Source: CAD feature listing. Evaluate the final solid. Frame: model axes, mm. Face numbers are marked on the shaded views. A direction names the side the tool comes from. Round coordinates to 2 decimals unless told otherwise and drop trailing zeros. Loops run counter-clockwise (first coordinate to the right, second up) from the corner with the lowest first, then second, coordinate; pieces in that order, holes last. Notation, with made-up numbers: (75, -10) - (131, -10) arc R17 cw to (131, 12) - close; hole circle Ø7 at (60, 60.5). An arc over 180 degrees is marked (long way). Use CSV: the item, a comma, the result in double quotes. Start each with the question number.
from build123d import *

# Parameters (mm, degrees)
SKETCH1_R           = 15
SKETCH1_R_2         = 13
BOSS_EXTRUDE1_DEPTH = 13
SKETCH2_R           = 18
SKETCH2_R_2         = 13
BOSS_EXTRUDE2_DEPTH = 2
CHAMFER1_SIZE       = 1
SKETCH4_R           = 18
SKETCH4_R_2         = 16.05
BOSS_EXTRUDE3_DEPTH = 3.8


with BuildPart() as part:
    # Sketch1 → Boss-Extrude1 (new body)
    with BuildSketch(Plane.XY):
        Circle(SKETCH1_R)
        Circle(SKETCH1_R_2, mode=Mode.SUBTRACT)
    extrude(amount=BOSS_EXTRUDE1_DEPTH)

    # Sketch2 → Boss-Extrude2 (add)
    with BuildSketch(Plane.XY.offset(13)):
        Circle(SKETCH2_R)
        Circle(SKETCH2_R_2, mode=Mode.SUBTRACT)
    extrude(amount=BOSS_EXTRUDE2_DEPTH)

    # Chamfer1
    chamfer1_edges = [part.edges().sort_by_distance(p)[0] for p in [
        (-13, 0, 15),
    ]]
    chamfer(chamfer1_edges, length=CHAMFER1_SIZE)

    # Sketch4 → Boss-Extrude3 (add)
    with BuildSketch(Plane.XY.offset(15)):
        Circle(SKETCH4_R)
        with Locations(Location((0, 0, 0), (0, 0, 180))):
            Circle(SKETCH4_R_2, mode=Mode.SUBTRACT)
    extrude(amount=BOSS_EXTRUDE3_DEPTH)


solid = part.part
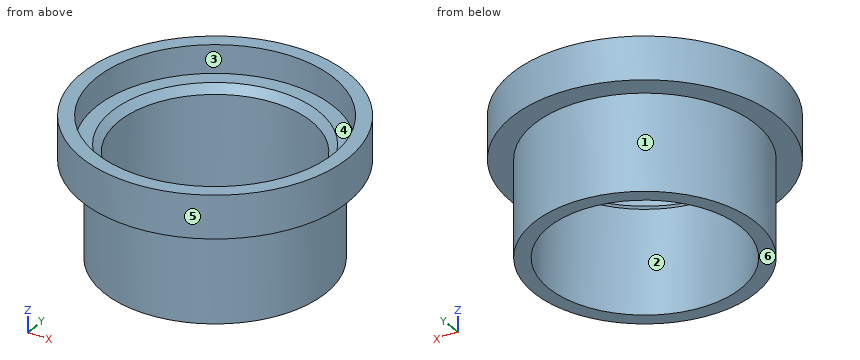
1. Section query C-C on z = 1.5. Return the cut outline in (x, y), and give its area (3 significant figures).
2. Contact query for flat-ended pins moving along their axis: P1, Ø10, axis at x = 12.5, y = -9, coming from the +Z side; P2, Ø2, axis at x = 1, z = 5, coming from the +Y side; P3, Ø1, axis at y = -5.5, z = 6.5, coming from the +X side; P4, Ø4, axis at y = -6.5, z = 10.5, coming from the -X side. Output: stop coordinate, or through.
3. Section query A-A on x = 0. Return the cut outline in (y, z).
4. Line query: line 1 along Y through (x, z) = (0, 7.5); line 2 along Y through (x, z) = (0, 17.15); line 3 along X through (y, z) = (-0.5, 12.5). Output: solid intervals per line, ascending.
5. Mould query, pull axis Y, two halves, no side actions, for the marked faces 4, 5 and 6. Classes: +Y half, -Y half, draft (parallel to the pull), parting line (faces both ways), or undercut.
6. Reachability of the marked faces 1, 2 and 3 from +Z, -Z, +X, -X, +Y, -Y: full face, straight path, thin tool, end or side. Return the list, or none.
Values:
1,outline,"circle Ø30 at (0, 0); hole circle Ø26 at (0, 0)"
1,area,"176 mm^2"
2,P1,"stops at z = 18.8"
2,P2,"stops at y = 15"
2,P3,"stops at x = 14.14"
2,P4,"stops at x = -14.31"
3,outline,"(-18, 13) - (-15, 13) - (-15, 0) - (-13, 0) - (-13, 14) - (-14, 15) - (-16.05, 15) - (-16.05, 18.8) - (-18, 18.8) - close; (13, 0) - (15, 0) - (15, 13) - (18, 13) - (18, 18.8) - (16.05, 18.8) - (16.05, 15) - (14, 15) - (13, 14) - close"
4,line 1,"y = -15 to -13, 13 to 15"
4,line 2,"y = -18 to -16.05, 16.05 to 18"
4,line 3,"x = -14.99 to -12.99, 12.99 to 14.99"
5,face 4,"undercut"
5,face 5,"parting line"
5,face 6,"draft"
6,face 1,"-Z"
6,face 2,"+Z, -Z"
6,face 3,"+Z"
